```python
from build123d import *

# Parameters (mm, degrees)
F0_R     = 21.75
F1_DEPTH = 90
F2_R     = 20.25
F3_DEPTH = 88
F5_DEPTH = 25
F7_DEPTH = 25


with BuildPart() as f1:
    # F0 (on Top) → F1 (new body)
    with BuildSketch(Plane.XY):
        Circle(F0_R)
    extrude(amount=F1_DEPTH)

    # F2 (on face) → F3 (cut)
    with BuildSketch(Plane.XY.offset(90)):
        Circle(F2_R)
    extrude(amount=-F3_DEPTH, mode=Mode.SUBTRACT)

    # F4 (on Right) → F5 (cut, symmetric)
    with BuildSketch(Plane.YZ):
        with BuildLine():
            Line((0, 11), (-1.299038, 8.75))
            ThreePointArc((-1.299038, 8.75), (0, 6.5), (1.299038, 8.75))
            Line((1.299038, 8.75), (0, 11))
        make_face()
    extrude(amount=F5_DEPTH, both=True, mode=Mode.SUBTRACT)

    # F6 (on Front) → F7 (cut, symmetric)
    with BuildSketch(Plane.XZ):
        with BuildLine():
            Line((0, 23), (-1.299038, 20.75))
            ThreePointArc((-1.299038, 20.75), (0, 18.5), (1.299038, 20.75))
            Line((1.299038, 20.75), (0, 23))
        make_face()
    extrude(amount=F7_DEPTH, both=True, mode=Mode.SUBTRACT)


solid = f1.part
```
Check sheet for the modelled part. Datum: model origin and axes. Units: mm. A direction names the side the tool comes from. Give positions to 0.01 mm unless a question says otherwise; leave off trailing zeros. Write each loop counter-clockwise with the first axis right and the second up, starting at its lowest first coordinate (ties: lowest second). Pieces come first, ordered by that corner, then holes. Notation, with made-up numbers: (-23, 13) - (-7, 13) arc R17 ccw to (-7, 36) - close; hole circle Ø3 at (-2, -7.5). An arc over 180 degrees is marked (long way). Answer as a JSON object with one key per item and string values. Group by question number.
1) Release check for a two-part mould opening along Z. For faces 3 (the face through (0, 21, 18.5)), 4 (the face through (0, 0, 0)), 5 (the face through (21, 0, 6.5)), 6 (the face through (0, 0, 2)) record: pulls with the +Z half, pulls with the -Z half, needs draft (parallel to the pull), parting line crosses it, or undercut.
2) Access from +Z, -Z, +X, -X, +Y, -Y to the whole of each face (thin tool, end or side, straight path). Record for faces 1 (the face through (-21, 0, 6.5)), 2 (the face through (19.315, 6.083, 46.616)).
3) Sectioned sample at A-A (x = -7). Record the cut outline in (y, z).
4) Thickness scan on probe 1 along X at (y, z) = (0, 61); probe 2 along Z at (x, y) = (-4, 11); probe 3 along Y at (x, z) = (16.5, 27.5). Record the ranges inside material, lowest first. Write a range as from..to.
5) Sectioned sample at C-C (y = -15.5). Record the cut outline in (x, z).
6) Depth check by flat-ended pin: P1, Ø2.5, axis at x = 0, z = 20, coming from the +Y side; P2, Ø1, axis at x = -2.5, y = 5, coming from the +Z side; P3, Ø4, axis at x = -16.5, z = 11, coming from the +Y side; P4, Ø2, axis at x = 10, z = 81, coming from the -Y side. Enter the tip coordinate at first touch or a pass-through.
7) Sectioned sample at B-B (z = 14.5). Record the cut outline in (x, y).
Geometry results:
{
 "1": {"face 3": "undercut", "face 4": "pulls with the -Z half", "face 5": "undercut", "face 6": "pulls with the +Z half"},
 "2": {"face 1": "+X, -X", "face 2": "+Z"},
 "3": {"outline": "(-20.59, 0) - (20.59, 0) - (20.59, 90) - (19, 90) - (19, 2) - (-19, 2) - (-19, 90) - (-20.59, 90) - close"},
 "4": {"probe 1": "x = -21.75..-20.25, 20.25..21.75", "probe 2": "z = 0..2", "probe 3": "y = -14.17..-11.74, 11.74..14.17"},
 "5": {"outline": "(-15.26, 0) - (15.26, 0) - (15.26, 90) - (13.03, 90) - (13.03, 2) - (-13.03, 2) - (-13.03, 90) - (-15.26, 90) - close"},
 "6": {"P1": "passes through", "P2": "stops at z = 2", "P3": "stops at y = 16.21", "P4": "stops at y = -19.8"},
 "7": {"outline": "circle Ø43.5 at (0, 0); hole circle Ø40.5 at (0, 0)"}
}
